The model under review builds one solid part; all positions refer to its coordinate system, in mm. A direction names the side the tool comes from. Round coordinates to 2 decimals unless told otherwise and drop trailing zeros. Write each loop counter-clockwise with the first axis right and the second up, starting at its lowest first coordinate (ties: lowest second). Pieces come first, ordered by that corner, then holes. Notation, with made-up numbers: (37, 79.25) -> (73, 79.25) arc R12 ccw to (73, 92.25) -> close; hole circle Ø6 at (57.25, 73.5). An arc over 180 degrees is marked (long way). Return JSON: item names as keys, results as strings. Group by question number.
1. Take a section at C-C, the plane y = 2.5. Write out the cut boundary in (x, z).
2. Tool access review of faces 5 (the flat face through (9, 5, 9)), 6 (the cylindrical face through (0.676, 2.465, 13.854)): name each direction out of +Z, -Z, +X, -X, +Y, -Y from which nothing blocks a thin tool from reaching the whole face with its end or side.
3. Clearance check with flat-ended pins moving along their axes: P1, Ø3, axis at y = 6, z = -2.5, coming from the -X side; P2, Ø2, axis at y = 11.5, z = 1, coming from the +X side; P3, Ø7, axis at x = 0, z = 16, coming from the -Y side; P4, Ø1, axis at y = 6.5, z = 5, coming from the +X side. State where each tip first meets the part, or that it passes through.
4. Take a section at B-B, the plane x = -16. Write out the cut boundary in (y, z).
5. Take a section at D-D, the plane x = 0. Write out the cut boundary in (y, z), then the cut area to 3 significant figures.
6. Take a section at A-A, the plane z = 16. Write out the cut boundary in (x, y).
7. For line 1 along Y through (x, z) = (9, -8.5); line 2 along X through (y, z) = (3.1, 16); line 3 along X through (y, z) = (13.25, -3), list the stretches that pass through material, from the lowest coordinate up. Write a range as from..to.
8. Mouldability with a two-part tool opening along X and no side actions: class faces 1 (the cylindrical face through (-19.524, 2.465, -4.336)), 2 (the flat face through (0, 0, 9)), 3 (the cylindrical face through (-7.81, 14.2, -1.73)), 4 (the cylindrical face through (-0.676, 2.465, -13.854)) as pulls with the +X half, pulls with the -X half, needs draft (parallel to the pull), parting line crosses it, or undercut.
from build123d import *

# Parameters (mm, degrees)
SKETCH_1_R          = 20
EXTRUDE_1_DEPTH     = 28
SKETCH_2_OUTSIDE_W  = 54.624
SKETCH_2_OUTSIDE_H  = 54.624
SKETCH_2_OUTSIDE_R  = 11
CUT_EXTRUDE_1_DEPTH = 23
SKETCH_3_R          = 8
CUT_EXTRUDE_2_DEPTH = 28
SKETCH_4_R          = 2.25
CUT_EXTRUDE_3_DEPTH = 5


with BuildPart() as part:
    # 草图1 → 凸台-拉伸1 (new body)
    with BuildSketch(Plane(origin=(0, 0, 0), x_dir=(1, 0, 0), z_dir=(0, 1, 0))):
        with Locations(Location((0, 0, 0), (0, 0, 270))):
            Circle(SKETCH_1_R)
    extrude(amount=EXTRUDE_1_DEPTH)

    # 草图2 outside → 切除-拉伸1 (cut)
    with BuildSketch(Plane(origin=(0, 28, 0), x_dir=(1, 0, 0), z_dir=(0, 1, 0))):
        Rectangle(SKETCH_2_OUTSIDE_W, SKETCH_2_OUTSIDE_H)
        with Locations(Location((0, 0, 0), (0, 0, 270))):
            Circle(SKETCH_2_OUTSIDE_R, mode=Mode.SUBTRACT)
    extrude(amount=-CUT_EXTRUDE_1_DEPTH, mode=Mode.SUBTRACT)

    # 草图3 → 切除-拉伸2 (cut)
    with BuildSketch(Plane(origin=(0, 28, 0), x_dir=(1, 0, 0), z_dir=(0, 1, 0))):
        with Locations(Location((0, 0, 0), (0, 0, 270))):
            Circle(SKETCH_3_R)
    extrude(amount=-CUT_EXTRUDE_2_DEPTH, mode=Mode.SUBTRACT)

    # 草图4 → 切除-拉伸3 (cut)
    with BuildSketch(Plane.XZ):
        with Locations(Location((0, 16, 0), (0, 0, 270))):
            Circle(SKETCH_4_R)
        with Locations(Location((16, 0, 0), (0, 0, 270))):
            Circle(SKETCH_4_R)
        with Locations(Location((0, -16, 0), (0, 0, 90))):
            Circle(SKETCH_4_R)
        with Locations(Location((-16, 0, 0), (0, 0, 90))):
            Circle(SKETCH_4_R)
    extrude(amount=-CUT_EXTRUDE_3_DEPTH, mode=Mode.SUBTRACT)


solid = part.part
Output:
{
 "1": {"outline": "circle Ø40 at (0, 0); hole circle Ø4.5 at (-16, 0); hole circle Ø16 at (0, 0); hole circle Ø4.5 at (0, -16); hole circle Ø4.5 at (0, 16); hole circle Ø4.5 at (16, 0)"},
 "2": {"face 5": "+Y", "face 6": "+Y, -Y"},
 "3": {"P1": "stops at x = -19.95", "P2": "stops at x = 11", "P3": "stops at y = 0", "P4": "stops at x = 10.04"},
 "4": {"outline": "(0, -12) -> (5, -12) -> (5, -2.25) -> (0, -2.25) -> close; (0, 2.25) -> (5, 2.25) -> (5, 12) -> (0, 12) -> close"},
 "5": {"outline": "(0, -20) -> (5, -20) -> (5, -18.25) -> (0, -18.25) -> close; (0, -13.75) -> (5, -13.75) -> (5, -11) -> (28, -11) -> (28, -8) -> (0, -8) -> close; (0, 8) -> (28, 8) -> (28, 11) -> (5, 11) -> (5, 13.75) -> (0, 13.75) -> close; (0, 18.25) -> (5, 18.25) -> (5, 20) -> (0, 20) -> close", "area": "213 mm^2"},
 "6": {"outline": "(-12, 0) -> (-2.25, 0) -> (-2.25, 5) -> (-12, 5) -> close; (2.25, 0) -> (12, 0) -> (12, 5) -> (2.25, 5) -> close"},
 "7": {"line 1": "y = 0..5", "line 2": "x = -12..-2.25, 2.25..12", "line 3": "x = -10.58..-7.42, 7.42..10.58"},
 "8": {"face 1": "parting line crosses it", "face 2": "needs draft", "face 3": "undercut", "face 4": "undercut"}
}
